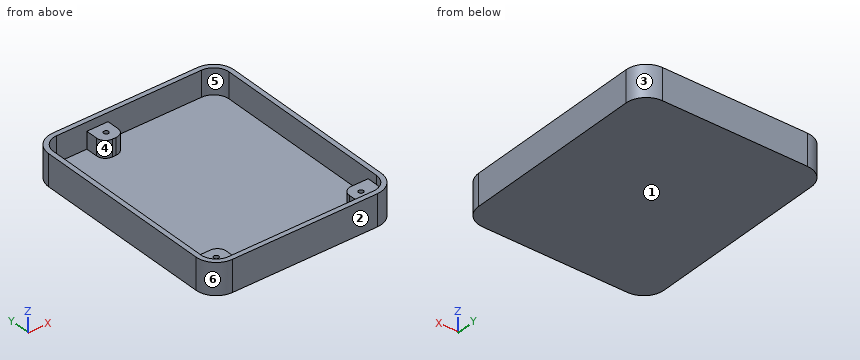
from build123d import *

# Parameters (mm, degrees)
EXTRUDE_1_DEPTH = 6.5
EXTRUDE_2_DEPTH = 1.2
SKETCH_4_R      = 0.5
EXTRUDE_3_DEPTH = 3.5


with BuildPart() as part:
    # Эскиз2 → Бобышка-Вытянуть1 (new body)
    with BuildSketch(Plane.XY):
        with BuildLine():
            Line((3.000001789, 45.2000009), (33.00000004, 45.2000009))
            ThreePointArc((33.00000004, 45.2000009), (35.969850924, 43.969847649), (37.20000166, 40.999995724))
            Line((37.20000166, 40.999995724), (37.20000166, 3.000004329))
            ThreePointArc((37.20000166, 3.000004329), (35.969850624, 0.030152951), (33.00000004, -1.2))
            Line((33.00000004, -1.2), (3.000001789, -1.2))
            ThreePointArc((3.000001789, -1.2), (0.030149154, 0.030152293), (-1.20000254, 3.000005176))
            Line((-1.20000254, 3.000005176), (-1.20000254, 40.999996571))
            ThreePointArc((-1.20000254, 40.999996571), (0.030149454, 43.969848906), (3.000001789, 45.2000009))
        make_face()
        with BuildLine():
            Line((3.000001789, 44.2000009), (33.00000004, 44.2000009))
            ThreePointArc((33.00000004, 44.2000009), (35.262743843, 43.262741167), (36.20000166, 40.999996571))
            Line((36.20000166, 40.999996571), (36.20000166, 3.000004329))
            ThreePointArc((36.20000166, 3.000004329), (35.262743843, 0.737259733), (33.00000004, -0.2))
            Line((33.00000004, -0.2), (3.000001789, -0.2))
            ThreePointArc((3.000001789, -0.2), (0.737256235, 0.737258775), (-0.20000254, 3.000004329))
            Line((-0.20000254, 3.000004329), (-0.20000254, 40.999996571))
            ThreePointArc((-0.20000254, 40.999996571), (0.737256235, 43.262742125), (3.000001789, 44.2000009))
        make_face(mode=Mode.SUBTRACT)
    extrude(amount=EXTRUDE_1_DEPTH)

    # Эскиз3 → Бобышка-Вытянуть2 (add)
    with BuildSketch(Plane.XY):
        with BuildLine():
            Line((-1.20000254, 40.999996571), (-1.20000254, 3.000005176))
            ThreePointArc((-1.20000254, 3.000005176), (0.030149154, 0.030152293), (3.000001789, -1.2))
            Line((3.000001789, -1.2), (33.00000004, -1.2))
            ThreePointArc((33.00000004, -1.2), (35.969850624, 0.030152951), (37.20000166, 3.000004329))
            Line((37.20000166, 3.000004329), (37.20000166, 40.999995724))
            ThreePointArc((37.20000166, 40.999995724), (35.969850924, 43.969847649), (33.00000004, 45.2000009))
            Line((33.00000004, 45.2000009), (3.000001789, 45.2000009))
            ThreePointArc((3.000001789, 45.2000009), (0.030149454, 43.969848906), (-1.20000254, 40.999996571))
        make_face()
    extrude(amount=EXTRUDE_2_DEPTH)

    # Эскиз4 → Бобышка-Вытянуть3 (add)
    # profile 1 of 3: a face of its own
    with BuildSketch(Plane.XY.offset(1.2)):
        with BuildLine():
            Line((9.271219031, 44.2000009), (13.669603576, 44.2000009))
            Line((13.669603576, 44.2000009), (13.669603576, 41.66326091))
            ThreePointArc((13.669603576, 41.66326091), (13.142395782, 40.390468704), (11.869603576, 39.86326091))
            Line((11.869603576, 39.86326091), (11.071219031, 39.86326091))
            ThreePointArc((11.071219031, 39.86326091), (9.798426825, 40.390468704), (9.271219031, 41.66326091))
            Line((9.271219031, 41.66326091), (9.271219031, 44.2000009))
        make_face()
        with Locations((11.49999986, 41.99999982)):
            Circle(SKETCH_4_R, mode=Mode.SUBTRACT)
    # profile 2 of 3: a face of its own
    with BuildSketch(Plane.XY.offset(1.2)):
        with BuildLine():
            Line((-0.20000254, 3.000004329), (-0.20000254, 5.158126066))
            Line((-0.20000254, 5.158126066), (3.542071928, 5.158126066))
            ThreePointArc((3.542071928, 5.158126066), (4.814864134, 4.630918272), (5.342071928, 3.358126066))
            Line((5.342071928, 3.358126066), (5.342071928, -0.2))
            Line((5.342071928, -0.2), (3.000001789, -0.2))
            ThreePointArc((3.000001789, -0.2), (0.737256235, 0.737258775), (-0.20000254, 3.000004329))
        make_face()
        with Locations((2.99999908, 3.00000162)):
            Circle(SKETCH_4_R, mode=Mode.SUBTRACT)
    # profile 3 of 3: a face of its own
    with BuildSketch(Plane.XY.offset(1.2)):
        with BuildLine():
            Line((33.00000004, -0.2), (30.851118491, -0.2))
            Line((30.851118491, -0.2), (30.851118491, 3.337368367))
            ThreePointArc((30.851118491, 3.337368367), (31.378326285, 4.610160574), (32.651118491, 5.137368367))
            Line((32.651118491, 5.137368367), (36.20000166, 5.137368367))
            Line((36.20000166, 5.137368367), (36.20000166, 3.000004329))
            ThreePointArc((36.20000166, 3.000004329), (35.262743843, 0.737259733), (33.00000004, -0.2))
        make_face()
        with Locations((33.00000004, 3.00000162)):
            Circle(SKETCH_4_R, mode=Mode.SUBTRACT)
    extrude(amount=EXTRUDE_3_DEPTH)


solid = part.part
Source: CAD feature listing. Evaluate the final solid. Frame: model axes, mm. Face numbers are marked on the shaded views. A direction names the side the tool comes from. Give positions to 0.01 mm unless a question says otherwise; leave off trailing zeros. Write each loop counter-clockwise with the first axis right and the second up, starting at its lowest first coordinate (ties: lowest second). Pieces come first, ordered by that corner, then holes. Notation, with made-up numbers: M -27,24.5 L 23,24.5 A9 ccw 23,34.5 Z; hole C 7,-19 d2. An arc over 180 degrees is marked long. Answer as a JSON object with one key per item and string values.
Q1. Contact query for flat-ended pins moving along their axis: P1, Ø3, axis at y = 43.5, z = 3, coming from the -X side; P2, Ø3, axis at x = 7.5, y = 32, coming from the +Z side; P3, Ø5, axis at x = 11, y = 41, coming from the +Z side. Output: stop coordinate, or through.
Geometry check:
{"P1": "stops at x = -1.08", "P2": "stops at z = 1.2", "P3": "stops at z = 4.7"}
Q2. Cut plane C-C, the plane x = 25. Return the cut outline in (y, z).
Geometry check:
{"outline": "M -1.2,0 L 45.2,0 L 45.2,6.5 L 44.2,6.5 L 44.2,1.2 L -0.2,1.2 L -0.2,6.5 L -1.2,6.5 Z"}
Q3. Cut plane A-A, the plane z = 2.25. Count the separate pieces of the cut face and the enclosed holes in it, then the cut area to 3 significant figures.
Geometry check:
{"separate pieces": "1", "enclosed holes": "4", "area": "227 mm^2"}
Q4. Access query for the marked faces 5 and 6. Directions: +Z, -Z, +X, -X, +Y, -Y. A direction counts if a zero-diameter tool reaches every point of the face in a straight line with its end or side. Return the directions, or none.
Geometry check:
{"face 5": "+Z", "face 6": "+Z, -Z, -X, -Y"}
Q5. Ray query, line 1 along Y through (x, z) = (11.5, 2.85); line 2 along X through (y, z) = (39, 1.25); line 3 along Y through (x, z) = (8.5, 6). Return the intervals inside material, ascending.
Geometry check:
{"line 1": "y = -1.2 to -0.2, 39.86 to 41.5, 42.5 to 45.2", "line 2": "x = -1.2 to -0.2, 36.2 to 37.2", "line 3": "y = -1.2 to -0.2, 44.2 to 45.2"}
Q6. Mould query, pull axis Y, two halves, no side actions, for the marked faces 1, 2, 3 and 4. Classes: +Y half, -Y half, draft (parallel to the pull), parting line (faces both ways), or undercut.
Geometry check:
{"face 1": "draft", "face 2": "-Y half", "face 3": "+Y half", "face 4": "undercut"}
Q7. Cut plane B-B, the plane y = 10. Return the cut outline in (x, z), then the cut area to 3 significant figures.
Geometry check:
{"outline": "M -1.2,0 L 37.2,0 L 37.2,6.5 L 36.2,6.5 L 36.2,1.2 L -0.2,1.2 L -0.2,6.5 L -1.2,6.5 Z", "area": "56.7 mm^2"}
